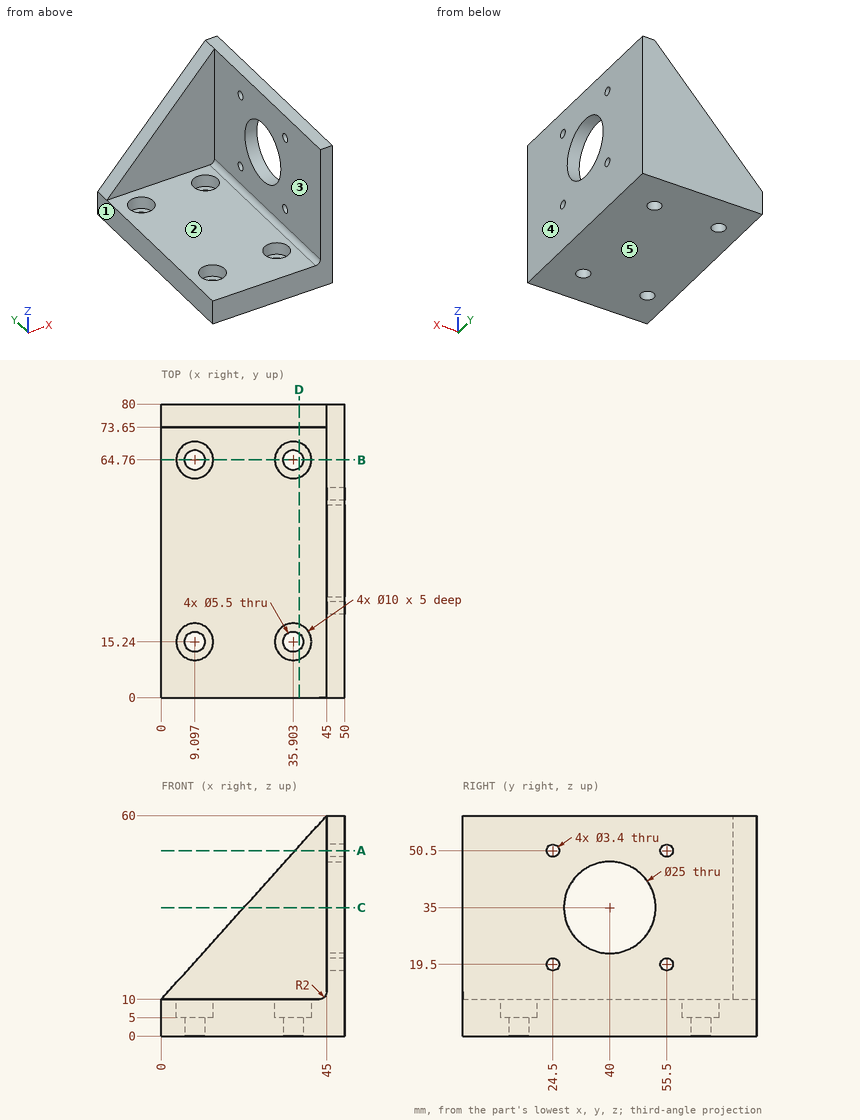
Study the drawing (mm; zero at the part's minimum x, y, z) and answer. A direction names the side the tool comes from. Coordinates: 2 decimals unless noted, no trailing zeros. Loops run counter-clockwise (first coordinate to the right, second up) from the corner with the lowest first, then second, coordinate; pieces in that order, holes last. Notation, with made-up numbers: (18, 8) -> (72, 8) arc R4 cw to (72, 14) -> close; hole circle Ø1 at (71, -14). An arc over 180 degrees is marked (long way). Answer in a Markdown table with one row per item. Add a question column.
1. The part is cut by section B-B, the plane y = 64.76. Write down the section's boundary in (x, z), then the cut area to 3 significant figures.
2. For the marked faces 1 and 2, determine the directions among +Z, -Z, +X, -X, +Y, -Y from which every point of the face is accessible in a straight line to the end or side of a thin tool.
3. The part is cut by section D-D, the plane x = 37.5. Write down the section's boundary in (y, z).
4. The part is cut by section A-A, the plane z = 50.5. Write down the section's boundary in (x, y), then the cut area to 3 significant figures.
5. The part is cut by section C-C, the plane z = 35. Write down the section's boundary in (x, y), then the cut area to 3 significant figures.
6. Determine the mould class of the marked faces 3, 4 and 5 for opening direction X: +X half, -X half, draft (parallel to the pull), parting line (faces both ways), or undercut.
7. Flat-ended cylindrical pins translate along their axes: P1, Ø3, axis at x = 36, y = 65.5, coming from the +Z side; P2, Ø9, axis at x = 9.1, y = 15.24, coming from the +Z side; P3, Ø2, axis at x = 30, y = 44.5, coming from the +Z side; P4, Ø6.5, axis at x = 35.9, y = 64.76, coming from the -Z side. Find the tip coordinate at first contact, or state that the pin passes through.
8. Consider line 1 (X direction, y = 64.76, z = 1.4); line 2 (X direction, y = 15, z = 6); line 3 (Y direction, x = 47.1, z = 50.5). Determine where each line is inside the solid, lowest interval first. Write a range as [from, to].
Answer below:
| question | item | result |
|---|---|---|
| 1 | outline | (0, 0) -> (6.35, 0) -> (6.35, 5) -> (4.1, 5) -> (4.1, 10) -> (0, 10) -> close; (11.85, 0) -> (33.15, 0) -> (33.15, 5) -> (30.9, 5) -> (30.9, 10) -> (14.1, 10) -> (14.1, 5) -> (11.85, 5) -> close; (38.65, 0) -> (50, 0) -> (50, 60) -> (45, 60) -> (45, 12) arc R2 cw to (43, 10) -> (40.9, 10) -> (40.9, 5) -> (38.65, 5) -> close |
| 1 | area | 596 mm2 |
| 2 | face 1 | +Z, -Z, -X, +Y, -Y |
| 2 | face 2 | +Z, -X, -Y |
| 3 | outline | (0, 0) -> (13, 0) -> (13, 5) -> (10.5, 5) -> (10.5, 10) -> (0, 10) -> close; (17.48, 0) -> (62.52, 0) -> (62.52, 5) -> (60.02, 5) -> (60.02, 10) -> (19.98, 10) -> (19.98, 5) -> (17.48, 5) -> close; (67, 0) -> (80, 0) -> (80, 51.67) -> (73.65, 51.67) -> (73.65, 10) -> (69.5, 10) -> (69.5, 5) -> (67, 5) -> close |
| 4 | outline | (36.45, 73.65) -> (45, 73.65) -> (45, 57.2) -> (50, 57.2) -> (50, 80) -> (36.45, 80) -> close; (45, 0) -> (50, 0) -> (50, 22.8) -> (45, 22.8) -> close; (45, 26.2) -> (50, 26.2) -> (50, 53.8) -> (45, 53.8) -> close |
| 4 | area | 420 mm2 |
| 5 | outline | (22.5, 73.65) -> (45, 73.65) -> (45, 52.5) -> (50, 52.5) -> (50, 80) -> (22.5, 80) -> close; (45, 0) -> (50, 0) -> (50, 27.5) -> (45, 27.5) -> close |
| 5 | area | 418 mm2 |
| 6 | face 3 | -X half |
| 6 | face 4 | +X half |
| 6 | face 5 | draft |
| 7 | P1 | through |
| 7 | P2 | z = 5 |
| 7 | P3 | z = 10 |
| 7 | P4 | z = 0 |
| 8 | line 1 | [0, 6.35], [11.85, 33.15], [38.65, 50] |
| 8 | line 2 | [0, 4.1], [14.09, 30.91], [40.9, 50] |
| 8 | line 3 | [0, 22.8], [26.2, 53.8], [57.2, 80] |
